For this review, use the dimensioned drawing (mm, ordinates from the lowest corner) and the shaded views. Coordinates: 2 decimals unless noted, no trailing zeros. Write each loop counter-clockwise with the first axis right and the second up, starting at its lowest first coordinate (ties: lowest second). Pieces come first, ordered by that corner, then holes. Notation, with made-up numbers: (75, 28) -> (124, 28) arc R27 cw to (124, 45) -> close; hole circle Ø9 at (4, 29). An arc over 180 degrees is marked (long way). Return JSON: item names as keys, results as strings. Group by question number.
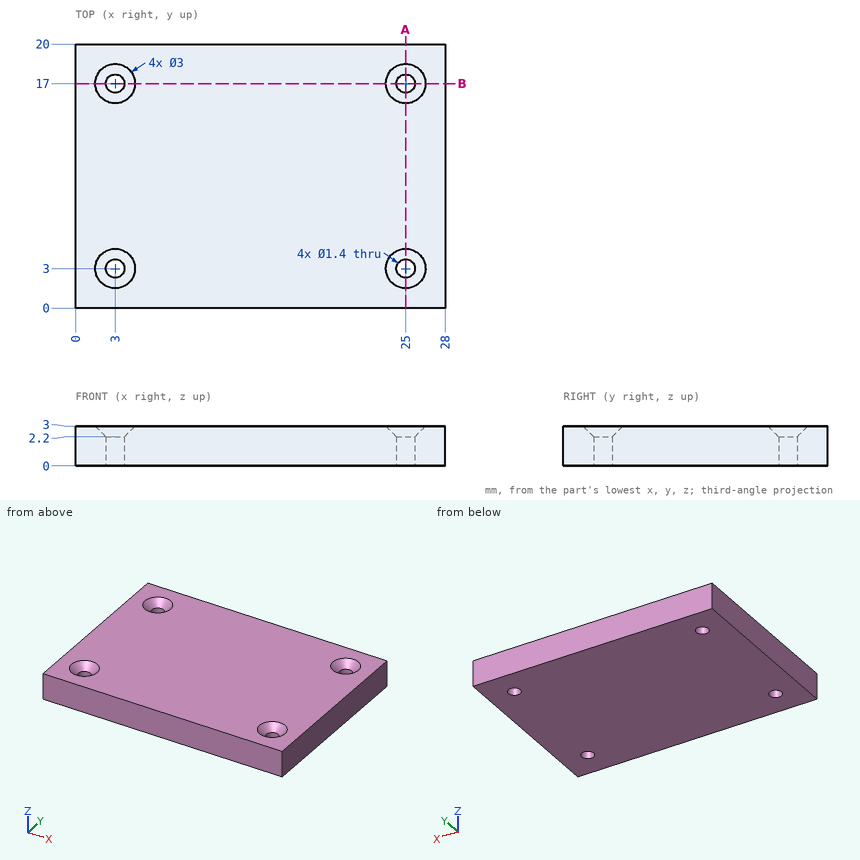
Q1. We need section A-A on x = 25. Write out the cut boundary in (y, z).
Q2. Wall thickness on L1, parallel to Y at x = 25, z = 0.8; L2, parallel to X at y = 3, z = 1.5; L3, parallel to X at y = 17.5, z = 0.65: over which ranges is each line inside the solid? List them lowest first.
Q3. We need section B-B on y = 17. Write out the cut boundary in (x, z), plus the area to 3 significant figures.
Q4. For P1, Ø1.3, axis at x = 3, y = 17, coming from the +Z side, flat-tipped, find the tip position at first contact; note if it passes through.
Findings below:
{
 "1": {"outline": "(0, 0) -> (2.3, 0) -> (2.3, 2.2) -> (1.5, 3) -> (0, 3) -> close; (3.7, 0) -> (16.3, 0) -> (16.3, 2.2) -> (15.5, 3) -> (4.5, 3) -> (3.7, 2.2) -> close; (17.7, 0) -> (20, 0) -> (20, 3) -> (18.5, 3) -> (17.7, 2.2) -> close"},
 "2": {"L1": "y = 0 to 2.3, 3.7 to 16.3, 17.7 to 20", "L2": "x = 0 to 2.3, 3.7 to 24.3, 25.7 to 28", "L3": "x = 0 to 2.51, 3.49 to 24.51, 25.49 to 28"},
 "3": {"outline": "(0, 0) -> (2.3, 0) -> (2.3, 2.2) -> (1.5, 3) -> (0, 3) -> close; (3.7, 0) -> (24.3, 0) -> (24.3, 2.2) -> (23.5, 3) -> (4.5, 3) -> (3.7, 2.2) -> close; (25.7, 0) -> (28, 0) -> (28, 3) -> (26.5, 3) -> (25.7, 2.2) -> close", "area": "74.3 mm^2"},
 "4": {"P1": "passes through"}
}
